```python
from build123d import *
from OCP.BRepFilletAPI import BRepFilletAPI_MakeFillet

# Parameters (mm, degrees)
ESQUISSE1_R        = 3
BOSS_EXTRU_1_DEPTH = 15
CONG_1_R1          = 50
CONG_1_R2          = 5


with BuildPart() as part:
    # Esquisse1 → Boss.-Extru.1 (new body)
    with BuildSketch(Plane.XY):
        Polygon((-450, 0), (-450, 20), (-420, 20), (-420, 70), (-405, 70), (-405, 20), (-85, 20), (-85, 70), (-70, 70), (-70, 20), (-50, 20), (-50, 0), (0, 0), (0, 100), (-100, 200), (-100, 250), (-85, 250), (-85, 300), (-100, 300), (-100, 350), (-85, 350), (-85, 400), (-100, 400), (-100, 450), (-85, 450), (-85, 500), (-100, 500), (-100, 550), (-85, 550), (-85, 600), (-100, 600), (-100, 650), (-85, 650), (-85, 700), (-100, 700), (-100, 750), (-85, 750), (-85, 800), (-100, 800), (-200, 800), (-500, 100), (-500, 0), align=None)
        with Locations((-412.5, 140)):
            Circle(ESQUISSE1_R, mode=Mode.SUBTRACT)
        with Locations((-77.5, 140)):
            Circle(ESQUISSE1_R, mode=Mode.SUBTRACT)
        Polygon((-180, 643.579383844), (-180, 140), (-395.819735933, 140), align=None, mode=Mode.SUBTRACT)
    extrude(amount=BOSS_EXTRU_1_DEPTH)

    # Congé1: one fillet with a radius per group of edges: ONE call of the kernel's fillet builder (fillet() takes one radius for all edges)
    cong_1_edges_1 = [part.edges().sort_by_distance(p)[0] for p in [
        (-200, 800, 7.5),
        (-180, 643.579383844, 7.5),
        (-395.819735933, 140, 7.5),
        (-180, 140, 7.5),
        (0, 100, 7.5),
        (-500, 100, 7.5),
    ]]
    cong_1_edges_2 = [part.edges().sort_by_distance(p)[0] for p in [
        (-85, 800, 7.5),
    ]]
    cong_1 = BRepFilletAPI_MakeFillet(part.part.solid().wrapped)
    for e in cong_1_edges_1:
        cong_1.Add(CONG_1_R1, e.wrapped)
    for e in cong_1_edges_2:
        cong_1.Add(CONG_1_R2, e.wrapped)
    add(Compound.cast(cong_1.Shape()), mode=Mode.REPLACE)


solid = part.part
```
Verification items for the finished model (mm, model axes). A direction names the side the tool comes from. Coordinates: 2 decimals unless noted, no trailing zeros. Write each loop counter-clockwise with the first axis right and the second up, starting at its lowest first coordinate (ties: lowest second). Pieces come first, ordered by that corner, then holes. Notation, with made-up numbers: M 28,51 L 36,51 A17 cw 36,82 Z; hole C 84.5,-38 d6. An arc over 180 degrees is marked long. One line per item, written item: value.
Item 1: Gauge pin test, flat ends, axial feed: pin 1 Ø1 at (x, z) = (-410.5, 8.5) entering from -Y; pin 2 Ø5 at (y, z) = (300.5, 5.5) entering from +X; pin 3 Ø4.5 at (y, z) = (620, 8.5) entering from +X. Record the tip position at first contact, or that the pin passes through.
Check sheet entries:
pin 1: stops at y = 70
pin 2: stops at x = -85
pin 3: stops at x = -100
Item 2: Section check A-A, the plane x = -468.5. Record the boundary of the cut face in (y, z), plus the area to 3 significant figures.
Check sheet entries:
outline: M 0,0 L 173.5,0 L 173.5,15 L 0,15 Z
area: 2,600 mm^2
Item 3: Access from +Z, -Z, +X, -X, +Y, -Y to the whole of each face (thin tool, end or side, straight path). Record for faces 1 (the flat face through (-57, 157, 7)), 2 (the flat face through (-352.49, 444.19, 7.4)), 3 (the flat face through (-85, 575, 7)), 4 (the flat face through (-405, 45, 7)), 5 (the cylindrical face through (-195.036, 154.258, 7.605)).
Check sheet entries:
face 1: +Z, -Z, +X
face 2: +Z, -Z, -X, +Y
face 3: +Z, -Z, +X, +Y
face 4: +Z, -Z, -Y
face 5: +Z, -Z
Item 4: Scan lines: line 1 along Y through (x, z) = (-145, 1); line 2 along X through (y, z) = (341.5, 10); line 3 along Y through (x, z) = (-77.5, 4.75). Record each from-to range of solid material in increasing order.
Check sheet entries:
line 1: y = 20 to 800
line 2: x = -396.5 to -309.46, -180 to -100
line 3: y = 70 to 137, 143 to 177.5
Item 5: Section check C-C, the plane y = 640.5. Record the boundary of the cut face in (x, z).
Check sheet entries:
outline: M -268.36,0 L -100,0 L -100,15 L -268.36,15 Z
Item 6: Section check B-B, the plane z = 5.25. State how many separate pieces and enclosed holes the cut face has, plus the area to 3 significant figures.
Check sheet entries:
separate pieces: 1
enclosed holes: 3
area: 181,000 mm^2
